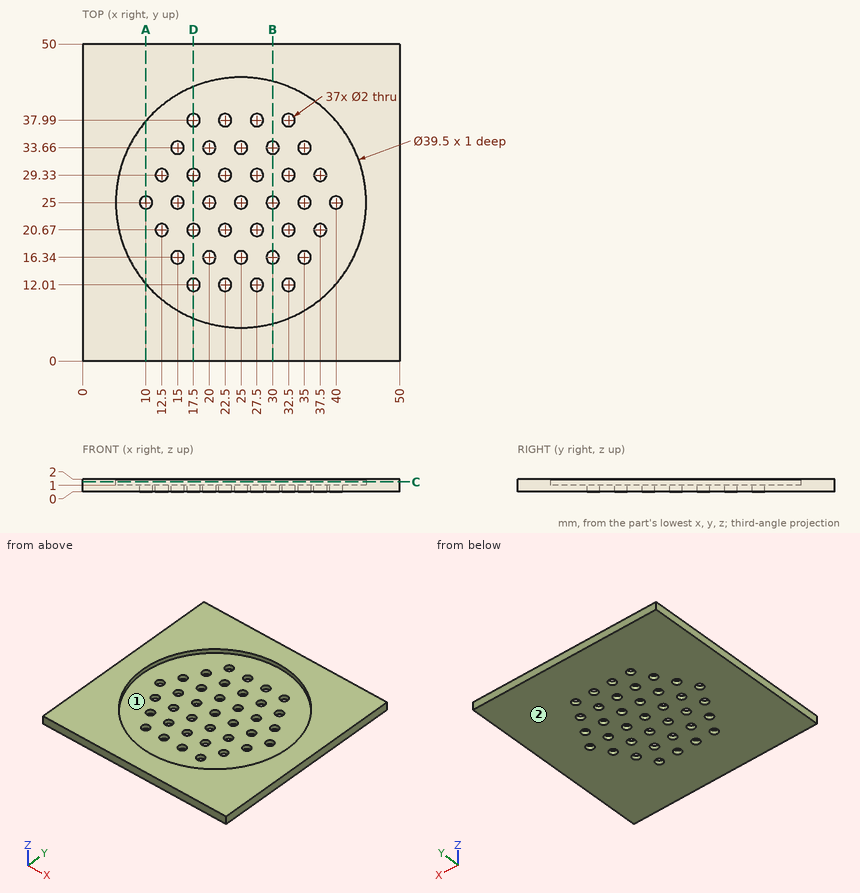
Geometry: see drawing. Coordinates: mm, zero at the bounding-box minimum. Round coordinates to 2 decimals unless told otherwise and drop trailing zeros. Loops run counter-clockwise (first coordinate to the right, second up) from the corner with the lowest first, then second, coordinate; pieces in that order, holes last. Notation, with made-up numbers: (27.5, 1) - (55.5, 1) arc R28 ccw to (55.5, 30) - close; hole circle Ø3 at (49, 86.5). An arc over 180 degrees is marked (long way). One line per item, written item: value. Start each with the question number.
(1) Draft query along X for the marked faces 1 and 2. Return one class per face: +X half, -X half, draft (parallel to the pull), parting line (faces both ways), or undercut.
(2) Section D-D, the plane x = 17.5. Return loops of the section in (y, z).
(3) Ray query, line 1 (Y direction, x = 20, z = 0.35); line 2 (Y direction, x = 27.5, z = 0.85); line 3 (Y direction, x = 12.5, z = 0.55). Return the intervals inside material, ascending. Write a range as [from, to].
(4) Section C-C, the plane z = 1.55. Return loops of the section in (x, y).
(5) Contact query for a flat-ended pin moving along its axis: P1, Ø2.5, axis at x = 22.5, y = 20.67, coming from the +Z side. Output: stop coordinate, or through.
(6) Section B-B, the plane x = 30. Return loops of the section in (y, z).
(7) Section A-A, the plane x = 10. Return loops of the section in (y, z).
Results below:
1. face 1: undercut
1. face 2: draft
2. outline: (0, 0) - (11.01, 0) - (11.01, 1) - (6.73, 1) - (6.73, 2) - (0, 2) - close; (13.01, 0) - (19.67, 0) - (19.67, 1) - (13.01, 1) - close; (21.67, 0) - (28.33, 0) - (28.33, 1) - (21.67, 1) - close; (30.33, 0) - (36.99, 0) - (36.99, 1) - (30.33, 1) - close; (38.99, 0) - (50, 0) - (50, 2) - (43.27, 2) - (43.27, 1) - (38.99, 1) - close
3. line 1: [0, 15.34], [17.34, 24], [26, 32.66], [34.66, 50]
3. line 2: [0, 11.01], [13.01, 19.67], [21.67, 28.33], [30.33, 36.99], [38.99, 50]
3. line 3: [0, 19.67], [21.67, 28.33], [30.33, 50]
4. outline: (0, 0) - (50, 0) - (50, 50) - (0, 50) - close; hole circle Ø39.5 at (25, 25)
5. P1: z = 1
6. outline: (0, 0) - (15.34, 0) - (15.34, 1) - (5.89, 1) - (5.89, 2) - (0, 2) - close; (17.34, 0) - (24, 0) - (24, 1) - (17.34, 1) - close; (26, 0) - (32.66, 0) - (32.66, 1) - (26, 1) - close; (34.66, 0) - (50, 0) - (50, 2) - (44.11, 2) - (44.11, 1) - (34.66, 1) - close
7. outline: (0, 0) - (24, 0) - (24, 1) - (12.15, 1) - (12.15, 2) - (0, 2) - close; (26, 0) - (50, 0) - (50, 2) - (37.85, 2) - (37.85, 1) - (26, 1) - close
